```python
from build123d import *

# Parameters (mm, degrees)
SKETCH1_W           = 42
SKETCH1_H           = 42
BOSS_EXTRUDE1_DEPTH = 11.5
CHAMFER1_SIZE       = 4
SKETCH2_R           = 11
BOSS_EXTRUDE2_DEPTH = 2
CUT_EXTRUDE1_START  = -0.5
SKETCH3_R           = 16
SKETCH3_R_2         = 11
CUT_EXTRUDE1_DEPTH  = 0.5
SKETCH4_R           = 2.5
BOSS_EXTRUDE3_DEPTH = 22
SKETCH5_W           = 10.364275964
SKETCH5_H           = 1.526028363
CUT_EXTRUDE2_DEPTH  = 20
CIRPATTERN1_COUNT   = 4
FILLET1_R           = 3
CHAMFER2_SIZE       = 0.5
FILLET2_R           = 1
FILLET3_R           = 0.5
SKETCH9_R           = 3.5
CUT_EXTRUDE3_DEPTH  = 3.5


with BuildPart() as part:
    # Sketch1 → Boss-Extrude1 (new, symmetric)
    with BuildSketch(Plane.XY):
        Rectangle(SKETCH1_W, SKETCH1_H)
    extrude(amount=BOSS_EXTRUDE1_DEPTH, both=True)

    # Chamfer1
    chamfer1_edges = [part.edges().sort_by_distance(p)[0] for p in [
        (21, -21, 0),
        (-21, -21, 0),
        (-21, 21, 0),
        (21, 21, 0),
    ]]
    chamfer(chamfer1_edges, length=CHAMFER1_SIZE)

    # Sketch2 → Boss-Extrude2 (add)
    with BuildSketch(Plane.XY.offset(11.5)):
        with Locations(Location((0, 0, 0), (0, 0, 180))):
            Circle(SKETCH2_R)
    extrude(amount=BOSS_EXTRUDE2_DEPTH)

    # Sketch3 → Cut-Extrude1 (cut)
    with BuildSketch(Plane.XY.offset(11.5).offset(CUT_EXTRUDE1_START)):
        Circle(SKETCH3_R)
        Circle(SKETCH3_R_2, mode=Mode.SUBTRACT)
    extrude(amount=CUT_EXTRUDE1_DEPTH, mode=Mode.SUBTRACT)

    # Sketch4 → Boss-Extrude3 (add)
    with BuildSketch(Plane.XY.offset(13.5)):
        Circle(SKETCH4_R)
    extrude(amount=BOSS_EXTRUDE3_DEPTH)

    # Sketch5 → Cut-Extrude2 (cut)
    with BuildSketch(Plane.XY.offset(35.5)):
        with Locations((0.738499094, 2.763014181)):
            Rectangle(SKETCH5_W, SKETCH5_H)
    extrude(amount=-CUT_EXTRUDE2_DEPTH, mode=Mode.SUBTRACT)

    # Sketch7 → M3x0.5 Tapped Hole1 (revolve, cut)
    with BuildSketch(Plane(origin=(-15.5, 15.5, 11.5), x_dir=(0, -1, 0), z_dir=(1, 0, 0))):
        Polygon((0, 0), (0, 8.251075774), (1.25, 7.5), (1.25, 0), align=None)
    m3x0_5_tapped_hole1 = revolve(axis=Axis((-15.5, 15.5, 17.85), (0, 0, -1)), mode=Mode.SUBTRACT)

    # CirPattern1: M3x0.5 Tapped Hole1 ×4 about axis
    cirpattern1_axis = Axis((0, 0, 0), (0, 0, 1))
    for i in range(1, CIRPATTERN1_COUNT):
        add(m3x0_5_tapped_hole1.rotate(cirpattern1_axis, i * 360 / CIRPATTERN1_COUNT), mode=Mode.SUBTRACT)

    # Fillet1
    fillet1_edges = [part.edges().sort_by_distance(p)[0] for p in [
        (17, -21, 0),
        (-17, -21, 0),
        (-21, 17, 0),
        (-21, -17, 0),
        (21, 17, 0),
        (21, -17, 0),
        (17, 21, 0),
        (-17, 21, 0),
    ]]
    fillet(fillet1_edges, radius=FILLET1_R)

    # Chamfer2
    chamfer2_edges = [part.edges().sort_by_distance(p)[0] for p in [
        (-1.118033989, -2.236067977, 35.5),
        (11, 0, 13.5),
    ]]
    chamfer(chamfer2_edges, length=CHAMFER2_SIZE - 0.0001)  # a hair under: the kernel refuses the full size

    # Fillet2
    fillet2_edges = [part.edges().sort_by_distance(p)[0] for p in [
        (-19, -19, -11.5),
        (0, -21, -11.5),
        (-19, 19, -11.5),
        (0, 21, -11.5),
        (19, 19, -11.5),
        (21, 0, -11.5),
        (19, -19, -11.5),
        (-16.90540961, 20.771638598, -11.5),
        (-20.771638598, 16.90540961, -11.5),
        (16.90540961, 20.771638598, -11.5),
        (20.771638598, 16.90540961, -11.5),
        (20.771638598, -16.90540961, -11.5),
        (16.90540961, -20.771638598, -11.5),
        (-16.90540961, -20.771638598, -11.5),
        (-20.771638598, -16.90540961, -11.5),
        (-21, 0, -11.5),
    ]]
    fillet(fillet2_edges, radius=FILLET2_R)

    # Fillet3
    fillet3_edges = [part.edges().sort_by_distance(p)[0] for p in [
        (-20.771638598, 16.90540961, 11.5),
        (16.90540961, 20.771638598, 11.5),
        (20.771638598, 16.90540961, 11.5),
        (20.771638598, -16.90540961, 11.5),
        (16.90540961, -20.771638598, 11.5),
        (-16.90540961, -20.771638598, 11.5),
        (-20.771638598, -16.90540961, 11.5),
        (-21, 0, 11.5),
        (-19, -19, 11.5),
        (0, -21, 11.5),
        (19, -19, 11.5),
        (21, 0, 11.5),
        (19, 19, 11.5),
        (0, 21, 11.5),
        (-19, 19, 11.5),
        (-16.90540961, 20.771638598, 11.5),
    ]]
    fillet(fillet3_edges, radius=FILLET3_R)

    # Sketch9 → Cut-Extrude3 (cut)
    with BuildSketch(Plane(origin=(0, 0, -11.5), x_dir=(-1, 0, 0), z_dir=(0, 0, -1))):
        Circle(SKETCH9_R)
    extrude(amount=-CUT_EXTRUDE3_DEPTH, mode=Mode.SUBTRACT)


solid = part.part
```
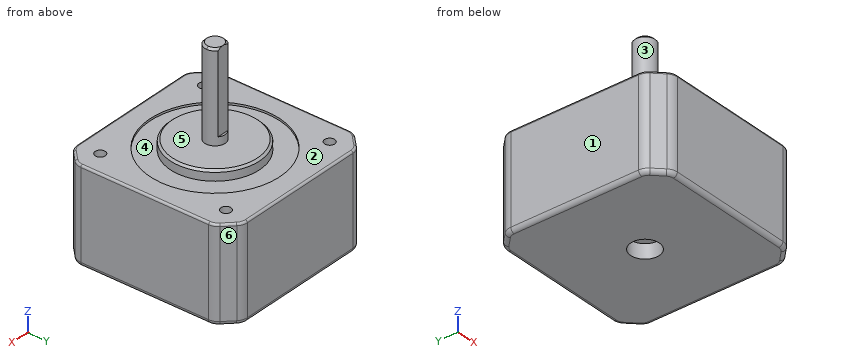
Input: part model. Units: mm. Frame: model coordinates. Face numbers are marked on the shaded views. A direction names the side the tool comes from. Give positions to 0.01 mm unless a question says otherwise; leave off trailing zeros. Write each loop counter-clockwise with the first axis right and the second up, starting at its lowest first coordinate (ties: lowest second). Pieces come first, ordered by that corner, then holes. Notation, with made-up numbers: (70.5, 24) - (103.5, 24) arc R29 ccw to (103.5, 52) - close; hole circle Ø5 at (37.5, 78.5). An arc over 180 degrees is marked (long way). Write item = value, one per line. Start each with the question number.
1. Ray query, L1, parallel to Y at x = -15.5, z = 8.75; L2, parallel to Y at x = -14.5, z = 7.5; L3, parallel to Y at x = 0, z = -9.9. Return the intervals inside material, ascending.
2. First-contact query: pin 1 Ø12 at (y, z) = (-5, 20) entering from +X; pin 2 Ø2 at (x, y) = (15.5, -15.5) entering from +Z; pin 3 Ø23 at (x, y) = (2.5, -3) entering from +Z; pin 4 Ø3 at (x, y) = (-15.5, -15.5) entering from +Z. Flat tips, straight axial feed; report the tip coordinate or a pass-through.
3. Section query A-A, the plane z = 7.5. Output: boundary loops of the cut face in (x, y).
4. Section query B-B, the plane z = 30. Output: boundary loops of the cut face in (x, y), then the cut area to 3 significant figures.
5. Mould query, pull axis X, two halves, no side actions, for the marked faces 1, 2, 3 and 4. Classes: released by +X, released by -X, zero draft, split by the parting line, or undercut.
6. Access query for the marked faces 5 and 6. Directions: +Z, -Z, +X, -X, +Y, -Y. A direction counts if a zero-diameter tool reaches every point of the face in a straight line with its end or side. Return the directions, or none.
Check sheet entries:
q1.L1 = -21 to -16.75, -14.25 to 14.25, 16.75 to 21
q1.L2 = -21 to -16.25, -14.75 to 14.75, 16.25 to 21
q1.L3 = -21 to -3.5, 3.5 to 21
q2.pin_1 = 2.5
q2.pin_2 = 3.85
q2.pin_3 = 35.5
q2.pin_4 = 11.5
q3.outline = (-21, -15.76) arc R3 ccw to (-20.12, -17.88) - (-17.88, -20.12) arc R3 ccw to (-15.76, -21) - (15.76, -21) arc R3 ccw to (17.88, -20.12) - (20.12, -17.88) arc R3 ccw to (21, -15.76) - (21, 15.76) arc R3 ccw to (20.12, 17.88) - (17.88, 20.12) arc R3 ccw to (15.76, 21) - (-15.76, 21) arc R3 ccw to (-17.88, 20.12) - (-20.12, 17.88) arc R3 ccw to (-21, 15.76) - close; hole circle Ø2.5 at (-15.5, -15.5); hole circle Ø2.5 at (-15.5, 15.5); hole circle Ø2.5 at (15.5, -15.5); hole circle Ø2.5 at (15.5, 15.5)
q4.outline = (-1.5, 2) arc R2.5 ccw (long way) to (1.5, 2) - close
q4.area = 18.6 mm2
q5.face_1 = released by -X
q5.face_2 = zero draft
q5.face_3 = split by the parting line
q5.face_4 = undercut
q6.face_5 = +Z
q6.face_6 = +Z, -Z, +X, +Y
